Could you check a few things on this model? Use its own coordinates, in mm. A direction names the side the tool comes from. Coordinates: 2 decimals unless noted, no trailing zeros. Write each loop counter-clockwise with the first axis right and the second up, starting at its lowest first coordinate (ties: lowest second). Pieces come first, ordered by that corner, then holes.
Item 1: I want a section at C-C on y = 42.5. Please give me the cut outline in (x, z).
Item 2: I want a section at B-B on x = -8. Please give me the cut outline in (y, z), then the cut area to 3 significant figures.
Item 3: I want a section at D-D on z = 97. Please give me the cut outline in (x, y).
Item 4: For P1, Ø4, axis at x = 2.5, z = 96.5, coming from the +Y side; P2, Ø5, axis at x = -10.5, z = 98, coming from the -Y side; P3, Ø2, axis at x = -8, z = 58, coming from the -Y side, each with a flat end and sliding along its axis, tell me the tip position at first contact or that it passes through.
Item 5: I want a section at A-A on z = 31. Please give me the cut outline in (x, y).
Item 6: If I drill on probe 1 along Y at (x, z) = (-6, 25); probe 2 along X at (y, z) = (-4, 6.5); probe 3 along Z at (x, y) = (0.5, -38), over which ranges is the centre line in solid material (lowest first)?
Item 7: Thinking about a two-plate mould opening in X: for faces 1 (the cylindrical face through (-14.985, 0.66, 59.16)), 2 (the flat face through (0, -60, 105)), 3 (the flat face through (-8.636, -5.043, 24.65)), which applies, +X half, -X half, draft (parallel to the pull), parting line (faces both ways), or undercut?
Item 8: Which directions (+Z, -Z, +X, -X, +Y, -Y) give clear straight access to the entire face, cutting with the end or side of a thin tool? Please do faces 4 (the flat face through (8.685, -4.958, 24.65)), 5 (the cylindrical face through (1.846, 36.533, 108.549)), 6 (the cylindrical face through (1.846, -35.924, 108.549)).
from build123d import *

# Parameters (mm, degrees)
CROQUIS2_R              = 15
SALIENTE_EXTRUIR1_DEPTH = 120
CORTAR_EXTRUIR1_DEPTH   = 50
CROQUIS4_R              = 4
SALIENTE_EXTRUIR2_DEPTH = 60
REDONDEO5_R             = 2


with BuildPart() as part:
    # Croquis2 → Saliente-Extruir1 (new body)
    with BuildSketch(Plane.XY):
        Circle(CROQUIS2_R)
    extrude(amount=SALIENTE_EXTRUIR1_DEPTH)

    # Croquis3 → Cortar-Extruir1 (cut)
    with BuildSketch(Plane(origin=(0, 0, 0), x_dir=(-1, 0, 0), z_dir=(0, 0, -1))):
        Polygon((5.741707523, 10.018289677), (-5.805239602, 9.981609414), (-11.546947124, -0.036680263), (-5.741707523, -10.018289677), (5.805239602, -9.981609414), (11.546947124, 0.036680263), align=None)
    extrude(amount=-CORTAR_EXTRUIR1_DEPTH, mode=Mode.SUBTRACT)

    # Croquis4 → Saliente-Extruir2 (add, symmetric)
    with BuildSketch(Plane(origin=(0, 0, 0), x_dir=(1, 0, 0), z_dir=(0, 1, 0))):
        with Locations((0, -105)):
            Circle(CROQUIS4_R)
    extrude(amount=SALIENTE_EXTRUIR2_DEPTH, both=True)

    # Redondeo5
    redondeo5_edges = [part.edges().sort_by_distance(p)[0] for p in [
        (-4, -60, 105),
        (-4, 60, 105),
    ]]
    fillet(redondeo5_edges, radius=REDONDEO5_R)


solid = part.part
Response values:
1. outline: circle Ø8 at (0, 105)
2. outline: (-12.69, 0) - (-6.15, 0) - (-6.15, 50) - (6.14, 50) - (6.14, 0) - (12.69, 0) - (12.69, 120) - (-12.69, 120) - close
2. area: 2,430 mm2
3. outline: circle Ø30 at (0, 0)
4. P1: stops at y = 14.99
4. P2: stops at y = -12.69
4. P3: stops at y = -13.27
5. outline: circle Ø30 at (0, 0); hole (-11.55, 0.04) - (-5.81, -9.98) - (5.74, -10.02) - (11.55, -0.04) - (5.81, 9.98) - (-5.74, 10.02) - close
6. probe 1: y = -13.75 to -9.64, 9.57 to 13.75
6. probe 2: x = -14.46 to -9.23, 9.24 to 14.46
6. probe 3: z = 101.03 to 108.97
7. face 1: parting line
7. face 2: draft
7. face 3: undercut
8. face 4: -Z
8. face 5: +Y
8. face 6: -Y
